Build history of the part. All positions in model axes, mm. A direction names the side the tool comes from. Round coordinates to 2 decimals unless told otherwise and drop trailing zeros. Order: outer loops, then holes, each group sorted by start corner. A loop starts at its lowest first (then second) coordinate and runs counter-clockwise, first axis right, second up. Notation, with made-up numbers: M 55.25,79.5 L 98.25,79.5 A12 cw 98.25,98.5 Z; hole C -24.5,3 d2. An arc over 180 degrees is marked long. One line per item, written item: value. Start each with the question number.
Item 1: Band-saw the part on C-C, the plane z = 33.25. Write the cut outline in (x, y).
Item 2: Band-saw the part on D-D, the plane x = 19. Write the cut outline in (y, z).
Item 3: Pin check, flat tips, straight feed: pin 1 (11 mm diameter, centred on x = 19.19, y = -32, fed in from +Z); pin 2 (1 mm diameter, centred on y = -27, z = 29.5, fed in from -X); pin 3 (3.5 mm diameter, centred on x = -4.5, z = 32.5, fed in from +Y); pin 4 (5 mm diameter, centred on x = -5.5, z = 32.5, fed in from +Y). Stop position of each tip, or through.
Item 4: Probe L1, parallel to Z at x = -3.5, y = -30.5; L2, parallel to X at y = -16, z = 34.5; L3, parallel to Y at x = -8, z = 35.5. List the from-to ranges inside material, lowest first.
Item 5: Tool access for faces 4 (the flat face through (2.209, -25, 29)), 5 (the flat face through (2.209, -45, 29)), 6 (the flat face through (0.1, -10, 33.1)): list every direction of +Z, -Z, +X, -X, +Y, -Y with a clear straight run to the whole face (end or side of a thin tool).
Item 6: Band-saw the part on A-A, the plane x = -5. Write the cut outline in (y, z), then the cut area to 3 significant figures.
Item 7: Band-saw the part on B-B, the plane y = -8. Write the cut outline in (x, z).
Item 8: Two-plate mould, pull along Z, no slides. Class faces 1 (the cylindrical face through (-4.33, -14.93, 38.47)), 2 (the flat face through (11, -25, 28.504)), 3 (the flat face through (0.1, -40, 33.1)): +Z half, -Z half, draft (parallel to the pull), parting line (faces both ways), or undercut.
```python
from build123d import *

# Parameters (mm, degrees)
F0_R     = 4
F1_DEPTH = 50
F2_R     = 3.5
F3_DEPTH = 2.001
F4_W     = 14.260426
F4_H     = 10
F4_W_2   = 14.935048
F4_W_3   = 15.686511
F5_DEPTH = 25


with BuildPart() as f1:
    # F0 (on Front) → F1 (new body)
    with BuildSketch(Plane.XZ):
        with BuildLine():
            Line((26.190159, 30.504479), (0.662295, 30.504479))
            ThreePointArc((0.662295, 30.504479), (-6.259331, 39.981705), (-3.809841, 28.504479))
            Line((-3.809841, 28.504479), (26.190159, 28.504479))
            Line((26.190159, 28.504479), (26.190159, 30.504479))
        make_face()
        with Locations((-3.809841, 34.504479)):
            Circle(F0_R, mode=Mode.SUBTRACT)
    extrude(amount=F1_DEPTH)

    # F2 (on face) → F3 (cut, through all)
    with BuildSketch(Plane.XY.offset(30.504479)):
        with Locations((19.190159, -32)):
            Circle(F2_R)
        with Locations((9.190159, -44)):
            Circle(F2_R)
        with Locations((9.190159, -20)):
            Circle(F2_R)
        with Locations((19.190159, -8)):
            Circle(F2_R)
    extrude(amount=-F3_DEPTH, mode=Mode.SUBTRACT)

    # F4 (on face) → F5 (cut)
    with BuildSketch(Plane(origin=(0, 0, 28.504479), x_dir=(1, 0, 0), z_dir=(0, 0, -1))):
        with Locations((-4.92115, 45)):
            Rectangle(F4_W, F4_H)
        with Locations((-5.258461, 25)):
            Rectangle(F4_W_2, F4_H)
        with Locations((-5.634192, 5)):
            Rectangle(F4_W_3, F4_H)
    extrude(amount=-F5_DEPTH, mode=Mode.SUBTRACT)


solid = f1.part
```
Output:
1. outline: M -9.68,-40 L -7.61,-40 L -7.61,-30 L -9.68,-30 Z; M -9.68,-20 L -7.61,-20 L -7.61,-10 L -9.68,-10 Z; M -0.01,-40 L 2.06,-40 L 2.06,-30 L -0.01,-30 Z; M -0.01,-20 L 2.06,-20 L 2.06,-10 L -0.01,-10 Z
2. outline: M -50,28.5 L -35.49,28.5 L -35.49,30.5 L -50,30.5 Z; M -28.51,28.5 L -11.49,28.5 L -11.49,30.5 L -28.51,30.5 Z; M -4.51,28.5 L 0,28.5 L 0,30.5 L -4.51,30.5 Z
3. pin 1: stops at z = 30.5
3. pin 2: stops at x = 2.21
3. pin 3: passes through
3. pin 4: stops at y = -10
4. L1: z = 28.5 to 30.52, 38.49 to 40.5
4. L2: x = -9.81 to -7.81, 0.19 to 2.19
4. L3: y = -40 to -30, -20 to -10
5. face 4: +Z, -Z, -X
5. face 5: +Z, -Z, -X, -Y
5. face 6: +Z, -Z, -X, +Y
6. outline: M -40,28.62 L -30,28.62 L -30,30.69 L -40,30.69 Z; M -40,38.32 L -30,38.32 L -30,40.39 L -40,40.39 Z; M -20,28.62 L -10,28.62 L -10,30.69 L -20,30.69 Z; M -20,38.32 L -10,38.32 L -10,40.39 L -20,40.39 Z
6. area: 82.5 mm²
7. outline: M 2.21,28.5 L 15.69,28.5 L 15.69,30.5 L 2.21,30.5 Z; M 22.69,28.5 L 26.19,28.5 L 26.19,30.5 L 22.69,30.5 Z
8. face 1: undercut
8. face 2: -Z half
8. face 3: draft
